Could you check a few things on this model? Use its own coordinates, in mm. A direction names the side the tool comes from. Round coordinates to 2 decimals unless told otherwise and drop trailing zeros. Write each loop counter-clockwise with the first axis right and the second up, starting at its lowest first coordinate (ties: lowest second). Pieces come first, ordered by that corner, then holes. Notation, with made-up numbers: (-36.75, 85) -> (19.25, 85) arc R18 ccw to (19.25, 89) -> close; hole circle Ø3 at (24, 22.5). An arc over 180 degrees is marked (long way). Answer in a Markdown table with one row per item.
from build123d import *

# Parameters (mm, degrees)
F1_DEPTH = 4.7752
F2_R     = 13.09751
F2_R_2   = 5.75437
F3_DEPTH = 25.4
F5_DEPTH = 25.4
F6_R     = 2.4638
F7_DEPTH = 25.4
F8_R     = 5.75437
F8_R_2   = 9.7282
F9_DEPTH = 25.4


with BuildPart() as f1:
    # F0 (on Right) → F1 (new body)
    with BuildSketch(Plane.YZ):
        Polygon((-304.8, 0), (0, 0), (304.8, 0), (304.8, 406.4), (0, 406.4), (-404.576362, 172.817728), align=None)
    extrude(amount=-F1_DEPTH)

    # F2 (on face) → F3 (cut)
    with BuildSketch(Plane.YZ):
        with Locations((218.948, 266.7)):
            Circle(F2_R)
        with Locations((184.023, 301.625)):
            Circle(F2_R_2)
        with Locations((253.873, 301.625)):
            Circle(F2_R_2)
        with Locations((253.873, 231.775)):
            Circle(F2_R_2)
        with Locations((184.023, 231.775)):
            Circle(F2_R_2)
        with Locations((63.5, 114.3)):
            Circle(F2_R_2)
        with Locations((241.3, 114.3)):
            Circle(F2_R_2)
        with Locations((241.3, 44.45)):
            Circle(F2_R_2)
        with Locations((63.5, 44.45)):
            Circle(F2_R_2)
        with Locations((152.4, 44.45)):
            Circle(F2_R_2)
    extrude(amount=-F3_DEPTH, mode=Mode.SUBTRACT)

    # F4 (on face) → F5 (cut)
    with BuildSketch(Plane.YZ):
        with BuildLine():
            ThreePointArc((176.529595, 383.243611), (139.227475, 361.707222), (111.540827, 328.71156))
            ThreePointArc((111.540827, 328.71156), (115.099736, 315.429531), (128.381765, 318.98844))
            ThreePointArc((128.381765, 318.98844), (151.727277, 346.810538), (183.180601, 364.970122))
            ThreePointArc((183.180601, 364.970122), (188.991842, 377.432369), (176.529595, 383.243611))
        make_face()
    extrude(amount=-F5_DEPTH, mode=Mode.SUBTRACT)

    # F6 (on face) → F7 (cut)
    with BuildSketch(Plane.YZ):
        with Locations((284.607, 25.4)):
            Circle(F6_R)
        with Locations((284.607, 76.2)):
            Circle(F6_R)
        with Locations((284.607, 127)):
            Circle(F6_R)
        with Locations((284.607, 381)):
            Circle(F6_R)
        with Locations((284.607, 177.8)):
            Circle(F6_R)
        with Locations((284.607, 228.6)):
            Circle(F6_R)
        with Locations((284.607, 279.4)):
            Circle(F6_R)
        with Locations((284.607, 330.2)):
            Circle(F6_R)
        with Locations((20.193, 25.4)):
            Circle(F6_R)
        with Locations((20.193, 330.2)):
            Circle(F6_R)
        with Locations((20.193, 76.2)):
            Circle(F6_R)
        with Locations((20.193, 127)):
            Circle(F6_R)
        with Locations((20.193, 177.8)):
            Circle(F6_R)
        with Locations((20.193, 228.6)):
            Circle(F6_R)
        with Locations((20.193, 279.4)):
            Circle(F6_R)
        with Locations((20.193, 381)):
            Circle(F6_R)
        with Locations((-374.388711, 160.917183)):
            Circle(F6_R)
        with Locations((-361.01303, 137.749824)):
            Circle(F6_R)
        with Locations((-313.38803, 55.260904)):
            Circle(F6_R)
        with Locations((-300.012349, 32.093545)):
            Circle(F6_R)
        with Locations((-337.20053, 96.505364)):
            Circle(F6_R)
    extrude(amount=-F7_DEPTH, mode=Mode.SUBTRACT)

    # F8 (on face) → F9 (cut)
    with BuildSketch(Plane.YZ):
        with Locations((-76.2, 114.3)):
            Circle(F8_R)
        with Locations((-76.2, 44.45)):
            Circle(F8_R)
        with Locations((-228.6, 114.3)):
            Circle(F8_R)
        with Locations((-228.6, 44.45)):
            Circle(F8_R)
        with Locations((-152.4, 254)):
            Circle(F8_R_2)
    extrude(amount=-F9_DEPTH, mode=Mode.SUBTRACT)


solid = f1.part
1) Imagine slicing it at A-A, the plane y = 225.5. Please give me the cut outline in (x, z), plus the area to 3 significant figures.
Findings:
| item | result |
|---|---|
| outline | (-4.78, 0) -> (0, 0) -> (0, 255.36) -> (-4.78, 255.36) -> close; (-4.78, 278.04) -> (0, 278.04) -> (0, 406.4) -> (-4.78, 406.4) -> close |
| area | 1,830 mm^2 |
2) Please list where these lines run through material, in increasing order: line 1 (Y direction, x = -1.5, z = 74); line 2 (Z direction, x = -0.6, y = 151.5); line 3 (Y direction, x = -0.5, z = 256).
Findings:
| item | result |
|---|---|
| line 1 | y = -347.52 to 19.08, 21.3 to 283.5, 285.72 to 304.8 |
| line 2 | z = 0 to 38.77, 50.13 to 346.62, 370.78 to 406.4 |
| line 3 | y = -260.5 to -161.92, -142.88 to 211.39, 226.5 to 304.8 |
3) Imagine slicing it at C-C, the plane y = -201.5. Please give me the cut outline in (x, z), plus the area to 3 significant figures.
Findings:
| item | result |
|---|---|
| outline | (-4.78, 0) -> (0, 0) -> (0, 290.06) -> (-4.78, 290.06) -> close |
| area | 1,390 mm^2 |
4) For faces 1 (the face through (-4.775, 24, 161)), 2 (the face through (-2.4, 139.7, 362.1)), which set-ups out of +Z, -Z, +X, -X, +Y, -Y let a thin tool reach every point of the face, with its end or its side?
Findings:
| item | result |
|---|---|
| face 1 | +Z, -Z, -X, +Y, -Y |
| face 2 | +X, -X |
5) Imagine slicing it at B-B, the plane x = -1. Count the separate pieces of the cut face and the enclosed holes in it, plus the area to 3 significant figures.
Findings:
| item | result |
|---|---|
| separate pieces | 1 |
| enclosed holes | 37 |
| area | 228,000 mm^2 |
6) Thinking about a two-plate mould opening in Z: for faces 3 (the face through (-2.354, 225.989, 277.744)), 4 (the face through (-2.354, -355.387, 87.619)), 5 (the face through (-2.35, -199.46, 291.24)), which applies, +Z half, -Z half, draft (parallel to the pull), parting line (faces both ways), or undercut?
Findings:
| item | result |
|---|---|
| face 3 | undercut |
| face 4 | -Z half |
| face 5 | +Z half |
